The model under review builds one solid part; all positions refer to its coordinate system, in mm. Coordinates: 2 decimals unless noted, no trailing zeros. Write each loop counter-clockwise with the first axis right and the second up, starting at its lowest first coordinate (ties: lowest second). Pieces come first, ordered by that corner, then holes.
1) Add section A-A, the plane x = -1.75. State the section outline as (y, z) points.
2) For line 1 (X direction, y = -0.95, z = 1.2); line 2 (Z direction, x = -8.75, y = 1.45); line 3 (X direction, y = 1.4, z = 0.95), list the stretches that pass through material, from the lowest coordinate up.
3) Mouldability with a two-part tool opening along X and no side actions: class faces 1 (the cylindrical face through (-2.45, 1.9, 0.08)), 2 (the cylindrical face through (-8, 0, -2)), 3 (the flat face through (0, 0, 0)) as released by +X, released by -X, zero draft, split by the parting line, or undercut.
from build123d import *

# Parameters (mm, degrees)
F0_R     = 2
F1_DEPTH = 2.2
F2_R     = 1.9
F3_DEPTH = 0.5
F4_R     = 2
F5_DEPTH = 10.8
F6_SIZE  = 0.5


with BuildPart() as f1:
    # F0 (on Right) → F1 (new body)
    with BuildSketch(Plane.YZ):
        Circle(F0_R)
    extrude(amount=-F1_DEPTH)

    # F2 (on face) → F3 (join)
    with BuildSketch(Plane(origin=(-2.2, 0, 0), x_dir=(0, -1, 0), z_dir=(-1, 0, 0))):
        Circle(F2_R)
    extrude(amount=F3_DEPTH)

    # F4 (on face) → F5 (join)
    with BuildSketch(Plane(origin=(-2.7, 0, 0), x_dir=(0, -1, 0), z_dir=(-1, 0, 0))):
        Circle(F4_R)
    extrude(amount=F5_DEPTH)

    # F6
    f6_edges = [f1.edges().sort_by_distance(p)[0] for p in [
        (0, -2, 0),
    ]]
    chamfer(f6_edges, length=F6_SIZE)


solid = f1.part
Geometry results:
1. outline: circle Ø4 at (0, 0)
2. line 1: x = -13.5 to -0.03
2. line 2: z = -1.38 to 1.38
2. line 3: x = -13.5 to -0.19
3. face 1: undercut
3. face 2: zero draft
3. face 3: released by +X
